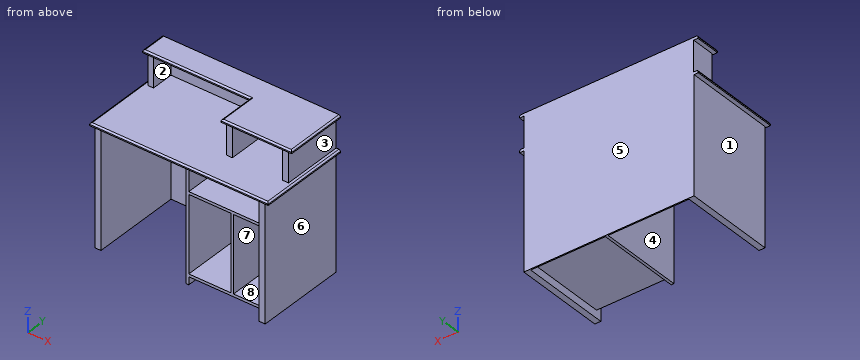
```python
from build123d import *

# Parameters (mm, degrees)
F0_W      = 18
F0_H      = 564
F1_DEPTH  = 780
F2_W      = 18
F2_H      = 512
F3_DEPTH  = 564
F5_DEPTH  = 18
F6_R      = 10
F7_W      = 40
F7_H      = 250
F7_H_2    = 150
F8_DEPTH  = 205
F10_DEPTH = 18
F11_R     = 10


with BuildPart() as f1:
    # F0 (on Top) → F1 (new body)
    with BuildSketch(Plane.XY):
        Polygon((-40, 0), (0, 0), (0, 608), (-1140, 608), (-1140, 0), (-1100, 0), (-1100, 600), (-558, 600), (-540, 600), (-40, 600), align=None)
        with Locations((-549, 318)):
            Rectangle(F0_W, F0_H)
    extrude(amount=F1_DEPTH)

    # F2 (on face) → F3 (join)
    with BuildSketch(Plane.XZ.offset(-600)):
        Polygon((-540, 70), (-540, 52), (-40, 52), (-40, 70), (-240, 70), (-258, 70), align=None)
        with Locations((-249, 326)):
            Rectangle(F2_W, F2_H)
        Polygon((-540, 582), (-258, 582), (-240, 582), (-40, 582), (-40, 600), (-540, 600), align=None)
    extrude(amount=F3_DEPTH)

    # F4 (on face) → F5 (join)
    with BuildSketch(Plane.XY.offset(780)):
        Polygon((28, 608), (0, 608), (-1140, 608), (-1168, 608), (-1168, -10), (28, -10), align=None)
    extrude(amount=F5_DEPTH)

    # F6
    f6_edges = [f1.edges().sort_by_distance(p)[0] for p in [
        (-570, -10, 798),
        (-1168, 299, 798),
        (28, 299, 798),
    ]]
    fillet(f6_edges, radius=F6_R)

    # F7 (on face) → F8 (join)
    with BuildSketch(Plane.XY.offset(798)):
        Polygon((-1100, 600), (-1100, 608), (-1137.470126, 608), (-1137.470126, 450), (-1100, 450), align=None)
        with Locations((-395.89883, 325)):
            Rectangle(F7_W, F7_H)
        with Locations((-395.89883, 525)):
            Rectangle(F7_W, F7_H_2)
        Polygon((0, 450), (0, 608), (-40, 608), (-40, 600), (-40, 450), align=None)
        with Locations((-20, 325)):
            Rectangle(F7_W, F7_H)
        Polygon((-40, 600), (-40, 608), (-1100, 608), (-1100, 600), (-415.89883, 600), (-375.89883, 600), align=None)
    extrude(amount=F8_DEPTH)

    # F9 (on face) → F10 (join)
    with BuildSketch(Plane.XY.offset(1003)):
        Polygon((0, 608), (-1137.470126, 608), (-1165.470126, 608), (-1165.470126, 440), (-443.89883, 440), (-443.89883, 190), (28, 190), (28, 608), align=None)
    extrude(amount=F10_DEPTH)

    # F11
    f11_edges = [f1.edges().sort_by_distance(p)[0] for p in [
        (-1165.470126, 524, 1021),
        (-804.684478, 440, 1021),
        (-443.89883, 315, 1021),
        (-207.949415, 190, 1021),
        (28, 399, 1021),
    ]]
    fillet(f11_edges, radius=F11_R)


solid = f1.part
```
The model under review builds one solid part; all positions refer to its coordinate system, in mm. Face numbers are marked on the shaded views. A direction names the side the tool comes from. Give positions to 0.01 mm unless a question says otherwise; leave off trailing zeros. Loops run counter-clockwise (first coordinate to the right, second up) from the corner with the lowest first, then second, coordinate; pieces in that order, holes last. Notation, with made-up numbers: (53, -1.75) -> (64, -1.75) arc R30 ccw to (64, 33.25) -> close; hole circle Ø5 at (40.5, -13.5). An arc over 180 degrees is marked (long way). Use CSV: the item, a comma, the result in double quotes.
1. Consider section B-B, the plane x = -466. Write out the cut boundary in (y, z).
Result:
outline,"(-10, 780) -> (600, 780) -> (600, 600) -> (36, 600) -> (36, 582) -> (600, 582) -> (600, 70) -> (36, 70) -> (36, 52) -> (600, 52) -> (600, 0) -> (608, 0) -> (608, 1021) -> (450, 1021) arc R10 ccw to (440, 1011) -> (440, 1003) -> (600, 1003) -> (600, 798) -> (0, 798) arc R10 ccw to (-10, 788) -> close"
2. Consider section A-A, the plane y = 54. Count the separate pieces of the cut face and the enclosed holes in it, then the cut area to 3 significant figures.
Result:
separate pieces,"1"
enclosed holes,"3"
area,"125,000 mm²"
3. To check wall thickness, follow probe 1 along X at (y, z) = (333, 332.5); probe 2 along Z at (x, y) = (-526, 41); probe 3 along X at (y, z) = (472, 880). State the ranges of each line that lie inside material, in increasing order. Write a range as from..to.
Result:
probe 1,"x = -1140..-1100, -558..-540, -258..-240, -40..0"
probe 2,"z = 52..70, 582..600, 780..798"
probe 3,"x = -1137.47..-1100, -415.9..-375.9, -40..0"
4. For P1, Ø1, axis at y = 412.5, z = 532, coming from the +X side; P2, Ø8, axis at x = -833.5, y = 413.5, coming from the +Z side; P3, Ø5, axis at x = -538.5, y = 545, coming from the -Z side; P4, Ø6.5, axis at y = 276, z = 1008.5, coming from the -X side, all flat-tipped, find the tip position at first contact; note any pin that passes through.
Result:
P1,"stops at x = 0"
P2,"stops at z = 798"
P3,"stops at z = 0"
P4,"stops at x = -443.9"
5. Consider section C-C, the plane z = 700.5. Write out the cut boundary in (x, y).
Result:
outline,"(-1140, 0) -> (-1100, 0) -> (-1100, 600) -> (-558, 600) -> (-558, 36) -> (-540, 36) -> (-540, 600) -> (-40, 600) -> (-40, 0) -> (0, 0) -> (0, 608) -> (-1140, 608) -> close"
6. The part is to be moulded in two halves that separate along X. For the marked faces 5, 6, 7 and 8, say which applies: +X half, -X half, draft (parallel to the pull), parting line (faces both ways), or undercut.
Result:
face 5,"draft"
face 6,"+X half"
face 7,"undercut"
face 8,"undercut"
7. Machinability: for the marked faces 1, 2, 3 and 4, which of the approach directions +Z, -Z, +X, -X, +Y, -Y give a long, thin tool a straight path to every point of the face, cutting with its end or side? Answer none if there is none.
Result:
face 1,"-Z, -X, +Y, -Y"
face 2,"-Y"
face 3,"+X, +Y, -Y"
face 4,"-Z, -Y"
